Design review of the part built by this model. Coordinates are the model's own, in mm. Face numbers are marked on the shaded views. Give positions to 0.01 mm unless a question says otherwise; leave off trailing zeros. Write each loop counter-clockwise with the first axis right and the second up, starting at its lowest first coordinate (ties: lowest second). Pieces come first, ordered by that corner, then holes. Notation, with made-up numbers: (-9, 19) - (27, 19) arc R14 ccw to (27, 44) - close; hole circle Ø4 at (-22, 64.25). An arc over 180 degrees is marked (long way). Use a Markdown table: item, result. Add a question column.
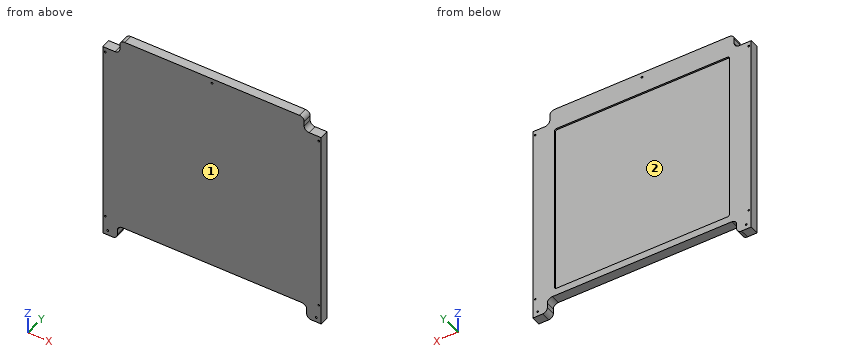
```python
from build123d import *

# Parameters (mm, degrees)
SKETCH2_W            = 450
SKETCH2_H            = 450
BOSS_EXTRUDE1_DEPTH  = 19.05
SKETCH7_W            = 35
SKETCH7_H            = 30
SKETCH7_W_2          = 390
CUT_EXTRUDE2_DEPTH   = 637.681162357
FILLET2_R            = 10
SKETCH3_W            = 360
SKETCH3_H            = 360
CUT_EXTRUDE1_DEPTH   = 3.175
FILLET1_R            = 3.175
M3_CLEARANCE_HOLE1_D = 3.6
M3_CLEARANCE_HOLE2_D = 3.6


with BuildPart() as part:
    # Sketch2 → Boss-Extrude1 (new body)
    with BuildSketch(Plane(origin=(0, 0, 0), x_dir=(1, 0, 0), z_dir=(0, 1, 0))):
        with Locations((225, 225)):
            Rectangle(SKETCH2_W, SKETCH2_H)
    extrude(amount=BOSS_EXTRUDE1_DEPTH)

    # Sketch7 → Cut-Extrude2 (cut, through all)
    with BuildSketch(Plane(origin=(0, 19.05, 0), x_dir=(1, 0, 0), z_dir=(0, 1, 0))):
        with Locations((432.5, 15)):
            Rectangle(SKETCH7_W, SKETCH7_H)
        with Locations((17.5, 15)):
            Rectangle(SKETCH7_W, SKETCH7_H)
        with Locations((225, 435)):
            Rectangle(SKETCH7_W_2, SKETCH7_H)
    extrude(amount=-CUT_EXTRUDE2_DEPTH, mode=Mode.SUBTRACT)

    # Fillet2
    fillet2_edges = [part.edges().sort_by_distance(p)[0] for p in [
        (35, 9.525, -30),
        (35, 9.525, 0),
        (30, 9.525, -420),
        (30, 9.525, -450),
        (420, 9.525, -450),
        (420, 9.525, -420),
        (415, 9.525, 0),
        (415, 9.525, -30),
    ]]
    fillet(fillet2_edges, radius=FILLET2_R)

    # Sketch3 → Cut-Extrude1 (cut)
    with BuildSketch(Plane(origin=(0, 19.05, 0), x_dir=(1, 0, 0), z_dir=(0, 1, 0))):
        with Locations((225, 225)):
            Rectangle(SKETCH3_W, SKETCH3_H)
    extrude(amount=-CUT_EXTRUDE1_DEPTH, mode=Mode.SUBTRACT)

    # Fillet1
    fillet1_edges = [part.edges().sort_by_distance(p)[0] for p in [
        (45, 17.4625, -405),
        (405, 17.4625, -405),
        (405, 17.4625, -45),
        (45, 17.4625, -45),
    ]]
    fillet(fillet1_edges, radius=FILLET1_R)

    # M3 Clearance Hole1 (through all)
    with Locations(Plane(origin=(440, 19.05, -440), x_dir=(0, 0, 1), z_dir=(0, 1, 0))):
        with Locations((0, 0), (0, -430), (430, -215)):
            Hole(M3_CLEARANCE_HOLE1_D / 2)

    # M3 Clearance Hole2 (through all)
    with Locations(Plane(origin=(445, 19.05, -410), x_dir=(0, 0, 1), z_dir=(0, 1, 0))):
        with Locations((0, 0), (0, -440), (370, -440), (370, 0)):
            Hole(M3_CLEARANCE_HOLE2_D / 2)


solid = part.part
```
(1) Add section A-A (y = 5.25). State the section outline as (x, z) points.
(2) Add section C-C (x = 389). State the section outline as (y, z) points (3 decimals).
(3) For line 1 along X through (y, z) = (4.25, -440); line 2 along Z through (x, y) = (445, 8.25); line 3 along X through (y, z) = (8.75, -40), list the stretches that pass through material, from the lowest coordinate up.
(4) Insertion check: pin 1 (6 mm diameter, centred on x = 225, z = -10, fed in from -Y); pin 2 (11 mm diameter, centred on y = 6, z = -17, fed in from +X); pin 3 (10 mm diameter, centred on x = 338, y = 2.5, fed in from -Z); pin 4 (3 mm diameter, centred on x = 5, z = -40, fed in from -Y). Each pin has a flat end and moves straight along its axis. Give the tip position at first contact, or say it passes through.
(5) Add section B-B (z = -199). State the section outline as (x, y) points (3 decimals), and give its area (3 significant figures).
(6) Mouldability with a two-part tool opening along X and no side actions: class the marked faces 1 and 2 as +X half, -X half, draft (parallel to the pull), parting line (faces both ways), or undercut.
Answers follow:
| question | item | result |
|---|---|---|
| 1 | outline | (0, -450) - (20, -450) arc R10 ccw to (30, -440) - (30, -430) arc R10 cw to (40, -420) - (410, -420) arc R10 cw to (420, -430) - (420, -440) arc R10 ccw to (430, -450) - (450, -450) - (450, -30) - (425, -30) arc R10 cw to (415, -20) - (415, -10) arc R10 ccw to (405, 0) - (45, 0) arc R10 ccw to (35, -10) - (35, -20) arc R10 cw to (25, -30) - (0, -30) - close; hole circle Ø3.6 at (5, -410); hole circle Ø3.6 at (5, -40); hole circle Ø3.6 at (10, -440); hole circle Ø3.6 at (225, -10); hole circle Ø3.6 at (440, -440); hole circle Ø3.6 at (445, -410); hole circle Ø3.6 at (445, -40) |
| 2 | outline | (0, -420) - (19.05, -420) - (19.05, -405) - (15.875, -405) - (15.875, -45) - (19.05, -45) - (19.05, 0) - (0, 0) - close |
| 3 | line 1 | 0 to 8.2, 11.8 to 30, 420 to 438.2, 441.8 to 450 |
| 3 | line 2 | -450 to -411.8, -408.2 to -41.8, -38.2 to -30 |
| 3 | line 3 | 0 to 3.2, 6.8 to 443.2, 446.8 to 450 |
| 4 | pin 1 | y = 0 |
| 4 | pin 2 | x = 415.32 |
| 4 | pin 3 | z = -420 |
| 4 | pin 4 | through |
| 5 | outline | (0, 0) - (450, 0) - (450, 19.05) - (405, 19.05) - (405, 15.875) - (45, 15.875) - (45, 19.05) - (0, 19.05) - close |
| 5 | area | 7,430 mm^2 |
| 6 | face 1 | draft |
| 6 | face 2 | undercut |
